Input: part model. Units: mm. Frame: model coordinates. Face numbers are marked on the shaded views. A direction names the side the tool comes from. Give positions to 0.01 mm unless a question says otherwise; leave off trailing zeros. Write each loop counter-clockwise with the first axis right and the second up, starting at its lowest first coordinate (ties: lowest second). Pieces come first, ordered by that corner, then holes. Notation, with made-up numbers: (69.25, 29.25) -> (84.25, 29.25) arc R11 cw to (84.25, 46.25) -> close; hole circle Ø8 at (66, 32.5). An arc over 180 degrees is marked (long way). Return JSON: item names as keys, results as strings. Group by question number.
Item 1: Section D-D, the plane x = 2.15. Return loops of the section in (y, z), then the cut area to 3 significant figures.
Item 2: Section A-A, the plane z = -4.5. Return loops of the section in (x, y).
Item 3: Section B-B, the plane x = -0.7. Return loops of the section in (y, z), then the cut area to 3 significant figures.
Item 4: Line query: line 1 (Y direction, x = -2.6, z = 3); line 2 (Z direction, x = 0.35, y = 0.65); line 3 (X direction, y = 0.35, z = -4.75). Output: solid intervals per line, ascending. Write a range as [from, to].
Item 5: Set-up query: the marked faces 1, 2 and 3. Return all of +Z, -Z, +X, -X, +Y, -Y with unobstructed straight access to the full face (end or side cutting, diameter ignored); none if empty.
Item 6: Section C-C, the plane y = 0.8. Return loops of the section in (x, z), then the cut area to 3 significant figures.
from build123d import *

# Parameters (mm, degrees)
SKETCH_1_W      = 2.6
SKETCH_1_H      = 9.6
EXTRUDE_1_DEPTH = 1.3
EXTRUDE_START   = 1.3
SKETCH_1_3_W    = 6
SKETCH_1_3_H    = 15
SKETCH_1_3_W_2  = 2.6
SKETCH_1_3_H_2  = 9.6
EXTRUDE_2_DEPTH = 2


with BuildPart() as part:
    # 草图1 → 凸台-拉伸1 (new body)
    with BuildSketch(Plane(origin=(0, 0, 0), x_dir=(1, 0, 0), z_dir=(0, 1, 0))):
        Rectangle(SKETCH_1_W, SKETCH_1_H)
    extrude(amount=EXTRUDE_1_DEPTH)

    # 草图1<3> → 凸台-拉伸2 (add)
    # profile 1 of 2: a face of its own
    with BuildSketch(Plane(origin=(0, 0, 0), x_dir=(1, 0, 0), z_dir=(0, 1, 0)).offset(EXTRUDE_START)):
        Rectangle(SKETCH_1_3_W, SKETCH_1_3_H)
        Rectangle(SKETCH_1_3_W_2, SKETCH_1_3_H_2, mode=Mode.SUBTRACT)
    # profile 2 of 2: a face of its own
    with BuildSketch(Plane(origin=(0, 0, 0), x_dir=(1, 0, 0), z_dir=(0, 1, 0)).offset(EXTRUDE_START)):
        Rectangle(SKETCH_1_3_W_2, SKETCH_1_3_H_2)
    extrude(amount=EXTRUDE_2_DEPTH)


solid = part.part
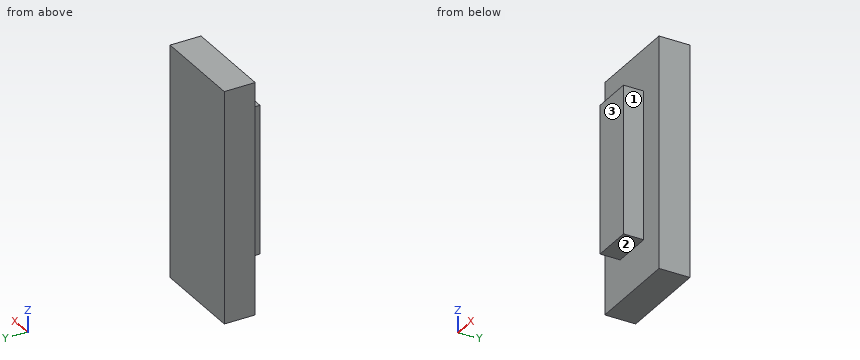
Answer below:
{
 "1": {"outline": "(1.3, -7.5) -> (3.3, -7.5) -> (3.3, 7.5) -> (1.3, 7.5) -> close", "area": "30.0 mm2"},
 "2": {"outline": "(-3, 1.3) -> (-1.3, 1.3) -> (-1.3, 0) -> (1.3, 0) -> (1.3, 1.3) -> (3, 1.3) -> (3, 3.3) -> (-3, 3.3) -> close"},
 "3": {"outline": "(0, -4.8) -> (1.3, -4.8) -> (1.3, -7.5) -> (3.3, -7.5) -> (3.3, 7.5) -> (1.3, 7.5) -> (1.3, 4.8) -> (0, 4.8) -> close", "area": "42.5 mm2"},
 "4": {"line 1": "y = [1.3, 3.3]", "line 2": "z = [-4.8, 4.8]", "line 3": "x = [-1.3, 1.3]"},
 "5": {"face 1": "+Z, -Z, +X, -Y", "face 2": "-Z, +X, -X, -Y", "face 3": "+Z, -Z, +X, -X, -Y"},
 "6": {"outline": "(-1.3, -4.8) -> (1.3, -4.8) -> (1.3, 4.8) -> (-1.3, 4.8) -> close", "area": "25.0 mm2"}
}
